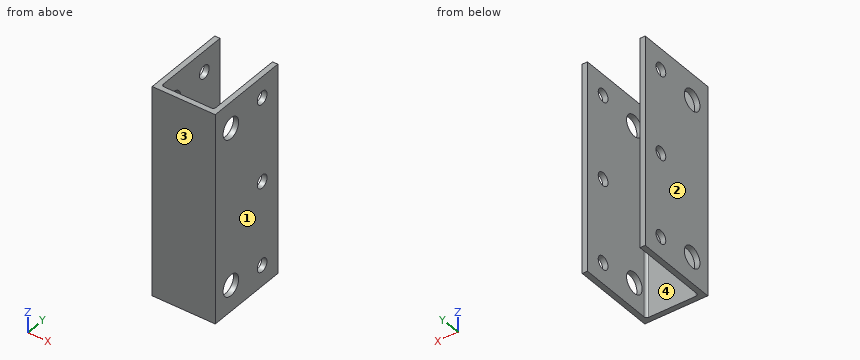
```python
from build123d import *

# Parameters (mm, degrees)
BOSS_EXTRUDE1_DEPTH = 127
SKETCH2_R           = 6.35
SKETCH2_R_2         = 3.96875
CUT_EXTRUDE1_DEPTH  = 152.4
FILLET1_R           = 1.6002


with BuildPart() as part:
    # Sketch1 → Boss-Extrude1 (new body)
    with BuildSketch(Plane.XY):
        Polygon((3.175, 50.8), (3.175, 3.175), (34.925, 3.175), (34.925, 50.8), (38.1, 50.8), (38.1, 0), (0, 0), (0, 50.8), align=None)
    extrude(amount=BOSS_EXTRUDE1_DEPTH)

    # Sketch2 → Cut-Extrude1 (cut)
    with BuildSketch(Plane(origin=(38.1, 0, 0), x_dir=(0, 0, -1), z_dir=(1, 0, 0))):
        with Locations((-15.875, 12.7)):
            Circle(SKETCH2_R)
        with Locations((-111.125, 12.7)):
            Circle(SKETCH2_R)
        with Locations((-114.3, 38.1)):
            Circle(SKETCH2_R_2)
        with Locations((-63.5, 38.1)):
            Circle(SKETCH2_R_2)
        with Locations((-12.7, 38.1)):
            Circle(SKETCH2_R_2)
    extrude(amount=-CUT_EXTRUDE1_DEPTH, mode=Mode.SUBTRACT)

    # Fillet1
    fillet1_edges = [part.edges().sort_by_distance(p)[0] for p in [
        (3.175, 3.175, 63.5),
        (34.925, 3.175, 63.5),
    ]]
    fillet(fillet1_edges, radius=FILLET1_R)


solid = part.part
```
Part model, mm, in its own coordinate system. Face numbers are marked on the shaded views. Coordinates: 2 decimals unless noted, no trailing zeros. Order: outer loops, then holes, each group sorted by start corner. A loop starts at its lowest first (then second) coordinate and runs counter-clockwise, first axis right, second up. Notation, with made-up numbers: (87, 4) - (125, 4) arc R8 ccw to (125, 9) - close; hole circle Ø6 at (60.25, 88). An arc over 180 degrees is marked (long way). Return JSON: item names as keys, results as strings. Group by question number.
Item 1: Drill centre lines: probe 1 along Z at (x, y) = (37, 38); probe 2 along X at (y, z) = (15, 69) (3 decimals); probe 3 along Z at (x, y) = (36.5, 37.5). Where is each one in solid material? Low to high. Write a range as from..to.
Item 2: Pin check, flat tips, straight feed: pin 1 (5 mm diameter, centred on x = 7, z = 71, fed in from +Y); pin 2 (7.5 mm diameter, centred on y = 12.7, z = 111.125, fed in from +X). Stop position of each tip, or through.
Item 3: Cut at D-D (y = 12.7). List the corners of the cut face in (x, z) (3 decimals), plus the area to 3 significant figures.
Item 4: Cut at B-B (z = 63.5). List the corners of the cut face in (x, y) (3 decimals), plus the area to 3 significant figures.
Item 5: Cut at C-C (y = 38.1). State how many separate pieces and enclosed holes the cut face has, plus the area to 3 significant figures.
Item 6: Pull direction X, two halves, no side cores. Call the marked faces 1, 2, 3 and 4: pulls with the +X half, pulls with the -X half, needs draft (parallel to the pull), parting line crosses it, or undercut.
Item 7: Cut at A-A (y = 46.5). List the corners of the cut face in (x, z) (3 decimals), plus the area to 3 significant figures.
Check values:
{
 "1": {"probe 1": "z = 0..8.73, 16.67..59.53, 67.47..110.33, 118.27..127", "probe 2": "x = 0..3.175, 34.925..38.1", "probe 3": "z = 0..8.78, 16.62..59.58, 67.42..110.38, 118.22..127"},
 "2": {"pin 1": "stops at y = 3.2", "pin 2": "passes through"},
 "3": {"outline": "(0, 0) - (3.175, 0) - (3.175, 9.525) - (0, 9.525) - close; (0, 22.225) - (3.175, 22.225) - (3.175, 104.775) - (0, 104.775) - close; (0, 117.475) - (3.175, 117.475) - (3.175, 127) - (0, 127) - close; (34.925, 0) - (38.1, 0) - (38.1, 9.525) - (34.925, 9.525) - close; (34.925, 22.225) - (38.1, 22.225) - (38.1, 104.775) - (34.925, 104.775) - close; (34.925, 117.475) - (38.1, 117.475) - (38.1, 127) - (34.925, 127) - close", "area": "645 mm2"},
 "4": {"outline": "(0, 0) - (38.1, 0) - (38.1, 34.131) - (34.925, 34.131) - (34.925, 4.775) arc R1.6 cw to (33.325, 3.175) - (4.775, 3.175) arc R1.6 cw to (3.175, 4.775) - (3.175, 34.131) - (0, 34.131) - close; (0, 42.069) - (3.175, 42.069) - (3.175, 50.8) - (0, 50.8) - close; (34.925, 42.069) - (38.1, 42.069) - (38.1, 50.8) - (34.925, 50.8) - close", "area": "374 mm2"},
 "5": {"separate pieces": "8", "enclosed holes": "0", "area": "655 mm2"},
 "6": {"face 1": "pulls with the +X half", "face 2": "pulls with the -X half", "face 3": "needs draft", "face 4": "undercut"},
 "7": {"outline": "(0, 0) - (3.175, 0) - (3.175, 127) - (0, 127) - close; (34.925, 0) - (38.1, 0) - (38.1, 127) - (34.925, 127) - close", "area": "806 mm2"}
}
